Input: dimensioned drawing with shaded views. Units: mm. Origin: part minimum x, y, z. Coordinates: 2 decimals unless noted, no trailing zeros. Order: outer loops, then holes, each group sorted by start corner. A loop starts at its lowest first (then second) coordinate and runs counter-clockwise, first axis right, second up. Notation, with made-up numbers: (-9, 52) -> (26, 52) arc R25 ccw to (26, 82) -> close; hole circle Ø6 at (20, 45.25). An arc over 180 degrees is marked (long way). Answer in a Markdown table with one row per item. Add a question column.
1) Section query C-C on x = 182. Return the cut outline in (y, z), then the cut area to 3 significant figures.
2) Ray query, line 1 (Y direction, x = 57.5, z = 0.6); line 2 (X direction, y = 62, z = 2.6) (1 decimal). Return the intervals inside material, ascending. Write a range as from..to.
3) Contact query for flat-ended pins moving along their axis: P1, Ø5, axis at x = 36.5, y = 56, coming from the +Z side; P2, Ø1.5, axis at y = 54.5, z = 1.5, coming from the -X side; P3, Ø1.5, axis at x = 1.5, z = 2, coming from the -Y side. Output: stop coordinate, or through.
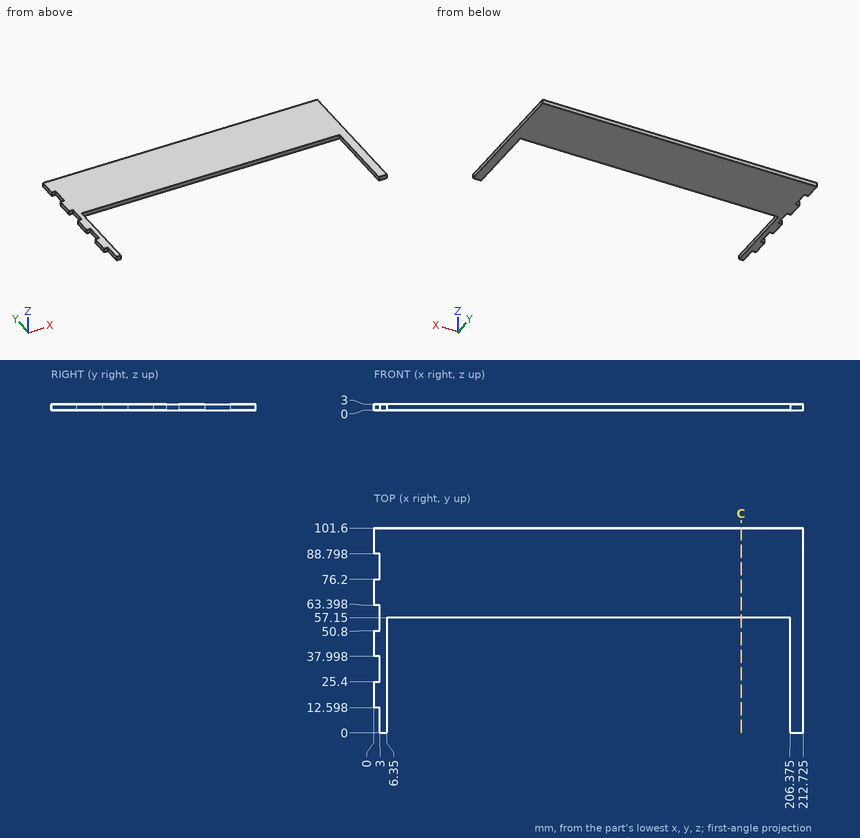
Result:
| question | item | result |
|---|---|---|
| 1 | outline | (57.15, 0) -> (101.6, 0) -> (101.6, 3) -> (57.15, 3) -> close |
| 1 | area | 133 mm2 |
| 2 | line 1 | 57.15..101.6 |
| 2 | line 2 | 3..212.7 |
| 3 | P1 | z = 3 |
| 3 | P2 | x = 3 |
| 3 | P3 | y = 12.6 |
